```python
from build123d import *

# Parameters (mm, degrees)
F1_DEPTH = 3
F3_DEPTH = 10
F4_R     = 1
F5_DEPTH = 5


with BuildPart() as f1:
    # F0 (on Top) → F1 (new body)
    with BuildSketch(Plane.XY):
        Polygon((5.7735026919, 10), (-5.7735026919, 10), (-11.5470053838, 0), (-5.7735026919, -10), (5.7735026919, -10), (11.5470053838, 0), align=None)
        with BuildLine():
            ThreePointArc((-3.3867513459, 4.1339745962), (-3.3867513459, 5.8660254038), (-1.8867513459, 5))
            Line((-1.8867513459, 5), (1.8867513459, 5))
            ThreePointArc((1.8867513459, 5), (2.8867513459, 6), (3.8867513459, 5))
            ThreePointArc((3.8867513459, 5), (3.7527767497, 4.5), (3.3867513459, 4.1339745962))
            Line((3.3867513459, 4.1339745962), (5.2735026919, 0.8660254038))
            ThreePointArc((5.2735026919, 0.8660254038), (6.2735026919, 0.8660254038), (6.7735026919, 0))
            ThreePointArc((6.7735026919, 0), (6.2735026919, -0.8660254038), (5.2735026919, -0.8660254038))
            Line((5.2735026919, -0.8660254038), (3.3867513459, -4.1339745962))
            ThreePointArc((3.3867513459, -4.1339745962), (3.7527767497, -4.5), (3.8867513459, -5))
            ThreePointArc((3.8867513459, -5), (2.8867513459, -6), (1.8867513459, -5))
            Line((1.8867513459, -5), (-1.8867513459, -5))
            ThreePointArc((-1.8867513459, -5), (-3.3867513459, -5.8660254038), (-3.3867513459, -4.1339745962))
            Line((-3.3867513459, -4.1339745962), (-5.2735026919, -0.8660254038))
            ThreePointArc((-5.2735026919, -0.8660254038), (-6.7735026919, 0), (-5.2735026919, 0.8660254038))
            Line((-5.2735026919, 0.8660254038), (-3.3867513459, 4.1339745962))
        make_face(mode=Mode.SUBTRACT)
        with BuildLine():
            Line((1.8867513459, 5), (-1.8867513459, 5))
            ThreePointArc((-1.8867513459, 5), (-2.3867513459, 4.1339745962), (-3.3867513459, 4.1339745962))
            Line((-3.3867513459, 4.1339745962), (-5.2735026919, 0.8660254038))
            ThreePointArc((-5.2735026919, 0.8660254038), (-4.9074772881, 0.5), (-4.7735026919, 0))
            ThreePointArc((-4.7735026919, 0), (-4.9074772881, -0.5), (-5.2735026919, -0.8660254038))
            Line((-5.2735026919, -0.8660254038), (-3.3867513459, -4.1339745962))
            ThreePointArc((-3.3867513459, -4.1339745962), (-2.3867513459, -4.1339745962), (-1.8867513459, -5))
            Line((-1.8867513459, -5), (1.8867513459, -5))
            ThreePointArc((1.8867513459, -5), (2.3867513459, -4.1339745962), (3.3867513459, -4.1339745962))
            Line((3.3867513459, -4.1339745962), (5.2735026919, -0.8660254038))
            ThreePointArc((5.2735026919, -0.8660254038), (4.7735026919, 0), (5.2735026919, 0.8660254038))
            Line((5.2735026919, 0.8660254038), (3.3867513459, 4.1339745962))
            ThreePointArc((3.3867513459, 4.1339745962), (2.3867513459, 4.1339745962), (1.8867513459, 5))
        make_face()
    extrude(amount=F1_DEPTH)

    # F2 (on face) → F3 (join)
    with BuildSketch(Plane.XY.offset(3)):
        Polygon((11.7779454915, 20.4), (-11.7779454915, 20.4), (-23.5558909829, 0), (-11.7779454915, -20.4), (11.7779454915, -20.4), (23.5558909829, 0), align=None)
        Polygon((5.7735026919, 10), (11.5470053838, 0), (5.7735026919, -10), (-5.7735026919, -10), (-11.5470053838, 0), (-5.7735026919, 10), align=None, mode=Mode.SUBTRACT)
        Polygon((11.7779454915, 20.4), (-11.7779454915, 20.4), (-23.5558909829, 0), (-11.7779454915, -20.4), (11.7779454915, -20.4), (23.5558909829, 0), align=None)
    extrude(amount=F3_DEPTH)

    # F4
    f4_edges = [f1.edges().sort_by_distance(p)[0] for p in [
        (-17.666918, 10.2, 13),
        (-17.666918, -10.2, 13),
        (0, -20.4, 13),
        (17.666918, -10.2, 13),
        (17.666918, 10.2, 13),
        (0, 20.4, 13),
        (-11.777945, 20.4, 8),
        (11.777945, 20.4, 8),
        (23.555891, 0, 8),
        (-23.555891, 0, 8),
        (11.777945, -20.4, 8),
        (-11.777945, -20.4, 8),
    ]]
    fillet(f4_edges, radius=F4_R)

    # F5 (cut): faces of the model
    f5_faces = [f1.faces().sort_by_distance(p)[0] for p in [
        (-2.8867513459, -5, 3),
        (2.8867513459, -5, 3),
        (5.7735026919, 0, 3),
        (2.8867513459, 5, 3),
        (-2.8867513459, 5, 3),
        (-5.7735026919, 0, 3),
    ]]
    extrude(f5_faces, amount=-F5_DEPTH, mode=Mode.SUBTRACT)


solid = f1.part
```
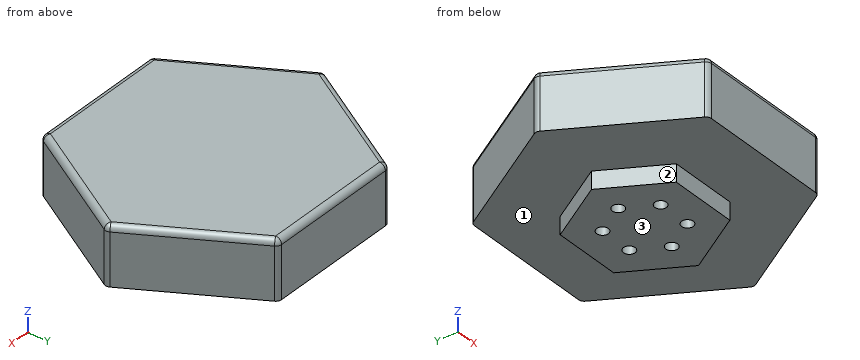
Could you check a few things on this model? Use its own coordinates, in mm. Face numbers are marked on the shaded views. A direction names the side the tool comes from. Coordinates: 2 decimals unless noted, no trailing zeros. Loops run counter-clockwise (first coordinate to the right, second up) from the corner with the lowest first, then second, coordinate; pieces in that order, holes last. Notation, with made-up numbers: M 71.25,8 L 106.25,8 A30 cw 106.25,44 Z; hole C -26.5,-37 d5. An arc over 180 degrees is marked long. Put each result on its own line as item: value. Start each with the question number.
(1) For the marked faces 1, 2 and 3, which set-ups out of +Z, -Z, +X, -X, +Y, -Y let a thin tool reach every point of the face, with its end or its side?
(2) Suppose I cut it at D-D on x = -7.5. Please give me the cut outline in (y, z), then the cut area to 3 significant figures.
(3) Suppose I cut it at A-A on z = 7. Please give me the cut outline in (x, y).
(4) Will these pins go through, and if not, where does the flat tip stop? P1, Ø5, axis at x = -14.5, z = 3.5, coming from the +Y side; P2, Ø8, axis at x = -2, y = -11, coming from the -Z side; P3, Ø1.5, axis at x = 0.5, z = 1, coming from the -Y side; P4, Ø0.6, axis at x = -2.5, y = 5, coming from the -Z side.
(5) Suppose I cut it at C-C on z = 2. Please give me the cut outline in (x, y).
(6) Suppose I cut it at B-B on x = 10. Please give me the cut outline in (y, z), then the cut area to 3 significant figures.
(7) I need wall thicknesses on line 1 (Y direction, x = 3, z = 7.25); line 2 (X direction, y = 5, z = 6.25); line 3 (Z direction, x = -5.5, y = 18). Which ranges of each line are inside material? Lowest first, please. Write a range as from..to.
Solutions:
1. face 1: -Z
1. face 2: -Z, -X, -Y
1. face 3: -Z, +X, -X, +Y, -Y
2. outline: M -20.4,3 L -7.01,3 L -7.01,0 L 7.01,0 L 7.01,3 L 20.4,3 L 20.4,12 A1 ccw 19.4,13 L -19.4,13 A1 ccw -20.4,12 Z
2. area: 450 mm2
3. outline: M -23.27,-0.5 L -12.07,-19.9 A1 ccw -11.2,-20.4 L 11.2,-20.4 A1 ccw 12.07,-19.9 L 23.27,-0.5 A1 ccw 23.27,0.5 L 12.07,19.9 A1 ccw 11.2,20.4 L -11.2,20.4 A1 ccw -12.07,19.9 L -23.27,0.5 A1 ccw Z; hole C -5.77,0 d2; hole C -2.89,-5 d2; hole C -2.89,5 d2; hole C 2.89,-5 d2; hole C 2.89,5 d2; hole C 5.77,0 d2
4. P1: stops at y = 20
4. P2: stops at z = 0
4. P3: stops at y = -10
4. P4: stops at z = 8
5. outline: M -11.55,0 L -5.77,-10 L 5.77,-10 L 11.55,0 L 5.77,10 L -5.77,10 Z; hole C -5.77,0 d2; hole C -2.89,-5 d2; hole C -2.89,5 d2; hole C 2.89,-5 d2; hole C 2.89,5 d2; hole C 5.77,0 d2
6. outline: M -20.4,3 L -2.68,3 L -2.68,0 L 2.68,0 L 2.68,3 L 20.4,3 L 20.4,12 A1 ccw 19.4,13 L -19.4,13 A1 ccw -20.4,12 Z
6. area: 424 mm2
7. line 1: y = -20.4..-5.99, -4.01..4.01, 5.99..20.4
7. line 2: x = -20.67..-3.89, -1.89..1.89, 3.89..20.67
7. line 3: z = 3..13
